Input: part model. Units: mm. Frame: model coordinates. A direction names the side the tool comes from. Round coordinates to 2 decimals unless told otherwise and drop trailing zeros. Write each loop counter-clockwise with the first axis right and the second up, starting at its lowest first coordinate (ties: lowest second). Pieces come first, ordered by that corner, then holes. Notation, with made-up numbers: (77.25, 14) - (92.25, 14) arc R20 ccw to (92.25, 31) - close; hole circle Ø9 at (19.5, -6). An arc over 180 degrees is marked (long way). One line per item, written item: value. Start each with the question number.
```python
from build123d import *

# Parameters (mm, degrees)
BOSS_EXTRUDE1_DEPTH = 25


with BuildPart() as part:
    # Sketch1 → Boss-Extrude1 (new, symmetric)
    with BuildSketch(Plane(origin=(0, 0, 0), x_dir=(0, 0, -1), z_dir=(1, 0, 0))):
        with BuildLine():
            Line((-60, 6.039014916), (60, 6.039014916))
            Line((60, 6.039014916), (60, 30.818764411))
            ThreePointArc((60, 30.818764411), (58.750354063, 32.039014916), (57.500708126, 30.818764411))
            Line((57.500708126, 30.818764411), (57.500708126, 11.039014916))
            ThreePointArc((57.500708126, 11.039014916), (55.57729196, 10.33874836), (53.653875793, 11.039014916))
            Line((53.653875793, 11.039014916), (53.653875793, 22.789014916))
            ThreePointArc((53.653875793, 22.789014916), (52.403875793, 24.039014916), (51.153875793, 22.789014916))
            Line((51.153875793, 22.789014916), (51.153875793, 11.039014916))
            ThreePointArc((51.153875793, 11.039014916), (49.049120778, 10.219058782), (46.944365764, 11.039014916))
            Line((46.944365764, 11.039014916), (46.944365764, 30.818764411))
            ThreePointArc((46.944365764, 30.818764411), (45.694719827, 32.039014916), (44.44507389, 30.818764411))
            Line((44.44507389, 30.818764411), (44.44507389, 11.039014916))
            ThreePointArc((44.44507389, 11.039014916), (42.521657723, 10.33874836), (40.598241557, 11.039014916))
            Line((40.598241557, 11.039014916), (40.598241557, 22.789014916))
            ThreePointArc((40.598241557, 22.789014916), (39.348241557, 24.039014916), (38.098241557, 22.789014916))
            Line((38.098241557, 22.789014916), (38.098241557, 11.039014916))
            ThreePointArc((38.098241557, 11.039014916), (35.993486542, 10.219058782), (33.888731528, 11.039014916))
            Line((33.888731528, 11.039014916), (33.888731528, 30.818764411))
            ThreePointArc((33.888731528, 30.818764411), (32.639085591, 32.039014916), (31.389439654, 30.818764411))
            Line((31.389439654, 30.818764411), (31.389439654, 11.039014916))
            ThreePointArc((31.389439654, 11.039014916), (29.466023487, 10.33874836), (27.54260732, 11.039014916))
            Line((27.54260732, 11.039014916), (27.54260732, 22.789014916))
            ThreePointArc((27.54260732, 22.789014916), (26.29260732, 24.039014916), (25.04260732, 22.789014916))
            Line((25.04260732, 22.789014916), (25.04260732, 11.039014916))
            ThreePointArc((25.04260732, 11.039014916), (22.937852306, 10.219058782), (20.833097291, 11.039014916))
            Line((20.833097291, 11.039014916), (20.833097291, 30.818764411))
            ThreePointArc((20.833097291, 30.818764411), (19.583451354, 32.039014916), (18.333805417, 30.818764411))
            Line((18.333805417, 30.818764411), (18.333805417, 11.039014916))
            ThreePointArc((18.333805417, 11.039014916), (16.410389251, 10.33874836), (14.486973084, 11.039014916))
            Line((14.486973084, 11.039014916), (14.486973084, 22.789014916))
            ThreePointArc((14.486973084, 22.789014916), (13.236973084, 24.039014916), (11.986973084, 22.789014916))
            Line((11.986973084, 22.789014916), (11.986973084, 11.039014916))
            ThreePointArc((11.986973084, 11.039014916), (9.88221807, 10.219058782), (7.777463055, 11.039014916))
            Line((7.777463055, 11.039014916), (7.777463055, 30.818764411))
            ThreePointArc((7.777463055, 30.818764411), (6.527817118, 32.039014916), (5.278171181, 30.818764411))
            Line((5.278171181, 30.818764411), (5.278171181, 11.039014916))
            ThreePointArc((5.278171181, 11.039014916), (3.354755015, 10.33874836), (1.431338848, 11.039014916))
            Line((1.431338848, 11.039014916), (1.431338848, 22.789014916))
            ThreePointArc((1.431338848, 22.789014916), (0.181338848, 24.039014916), (-1.068661152, 22.789014916))
            Line((-1.068661152, 22.789014916), (-1.068661152, 11.039014916))
            ThreePointArc((-1.068661152, 11.039014916), (-3.173416167, 10.219058782), (-5.278171181, 11.039014916))
            Line((-5.278171181, 11.039014916), (-5.278171181, 30.818764411))
            ThreePointArc((-5.278171181, 30.818764411), (-6.527817118, 32.039014916), (-7.777463055, 30.818764411))
            Line((-7.777463055, 30.818764411), (-7.777463055, 11.039014916))
            ThreePointArc((-7.777463055, 11.039014916), (-9.700879222, 10.33874836), (-11.624295388, 11.039014916))
            Line((-11.624295388, 11.039014916), (-11.624295388, 22.789014916))
            ThreePointArc((-11.624295388, 22.789014916), (-12.874295388, 24.039014916), (-14.124295388, 22.789014916))
            Line((-14.124295388, 22.789014916), (-14.124295388, 11.039014916))
            ThreePointArc((-14.124295388, 11.039014916), (-16.229050403, 10.219058782), (-18.333805417, 11.039014916))
            Line((-18.333805417, 11.039014916), (-18.333805417, 30.818764411))
            ThreePointArc((-18.333805417, 30.818764411), (-19.583451354, 32.039014916), (-20.833097291, 30.818764411))
            Line((-20.833097291, 30.818764411), (-20.833097291, 11.039014916))
            ThreePointArc((-20.833097291, 11.039014916), (-22.756513458, 10.33874836), (-24.679929625, 11.039014916))
            Line((-24.679929625, 11.039014916), (-24.679929625, 22.789014916))
            ThreePointArc((-24.679929625, 22.789014916), (-25.929929625, 24.039014916), (-27.179929625, 22.789014916))
            Line((-27.179929625, 22.789014916), (-27.179929625, 11.039014916))
            ThreePointArc((-27.179929625, 11.039014916), (-29.284684639, 10.219058782), (-31.389439654, 11.039014916))
            Line((-31.389439654, 11.039014916), (-31.389439654, 30.818764411))
            ThreePointArc((-31.389439654, 30.818764411), (-32.639085591, 32.039014916), (-33.888731528, 30.818764411))
            Line((-33.888731528, 30.818764411), (-33.888731528, 11.039014916))
            ThreePointArc((-33.888731528, 11.039014916), (-35.812147694, 10.33874836), (-37.735563861, 11.039014916))
            Line((-37.735563861, 11.039014916), (-37.735563861, 22.789014916))
            ThreePointArc((-37.735563861, 22.789014916), (-38.985563861, 24.039014916), (-40.235563861, 22.789014916))
            Line((-40.235563861, 22.789014916), (-40.235563861, 11.039014916))
            ThreePointArc((-40.235563861, 11.039014916), (-42.340318875, 10.219058782), (-44.44507389, 11.039014916))
            Line((-44.44507389, 11.039014916), (-44.44507389, 30.818764411))
            ThreePointArc((-44.44507389, 30.818764411), (-45.694719827, 32.039014916), (-46.944365764, 30.818764411))
            Line((-46.944365764, 30.818764411), (-46.944365764, 11.039014916))
            ThreePointArc((-46.944365764, 11.039014916), (-48.86778193, 10.33874836), (-50.791198097, 11.039014916))
            Line((-50.791198097, 11.039014916), (-50.791198097, 22.789014916))
            ThreePointArc((-50.791198097, 22.789014916), (-52.041198097, 24.039014916), (-53.291198097, 22.789014916))
            Line((-53.291198097, 22.789014916), (-53.291198097, 11.039014916))
            ThreePointArc((-53.291198097, 11.039014916), (-55.395953112, 10.219058782), (-57.500708126, 11.039014916))
            Line((-57.500708126, 11.039014916), (-57.500708126, 30.818764411))
            ThreePointArc((-57.500708126, 30.818764411), (-58.750354063, 32.039014916), (-60, 30.818764411))
            Line((-60, 30.818764411), (-60, 6.039014916))
        make_face()
    extrude(amount=BOSS_EXTRUDE1_DEPTH, both=True)


solid = part.part
```
Q1. Cut plane A-A, the plane y = 13.75. Count the separate pieces of the cut face and the enclosed holes in it, and give its area (3 significant figures).
Q2. Material intervals for probe 1 along Y at (x, z) = (-11, 35.5); probe 2 along Y at (x, z) = (-22, -39.5), sorted ascending. Write a range as from..to.
Q3. Access query for faces 1 (the flat face through (0, 17, -38.098)), 2 (the flat face through (25, 13.4, -12.5)). Directions: +Z, -Z, +X, -X, +Y, -Y. A direction counts if a zero-diameter tool reaches every point of the face in a straight line with its end or side. Return the directions, or none.
Q4. Cut plane D-D, the plane z = -29. Output: boundary loops of the cut face in (x, y).
Q5. Cut plane C-C, the plane z = -49.5. Output: boundary loops of the cut face in (x, y), and give its area (3 significant figures).
Q6. Pull-direction query (Z, two-part tool) for faces 3 (the flat face through (0, 17, 50.791)), 4 (the flat face through (0, 6.039, 1)); classes: pulls with the +Z half, pulls with the -Z half, needs draft (parallel to the pull), parting line crosses it, or undercut.
A:
1. separate pieces: 19
1. enclosed holes: 0
1. area: 2,370 mm²
2. probe 1: y = 6.04..10.36
2. probe 2: y = 6.04..24.03
3. face 1: +X, -X, +Y
3. face 2: +Z, -Z, +X, +Y, -Y
4. outline: (-25, 6.04) - (25, 6.04) - (25, 10.38) - (-25, 10.38) - close
5. outline: (-25, 6.04) - (25, 6.04) - (25, 10.25) - (-25, 10.25) - close
5. area: 211 mm²
6. face 3: undercut
6. face 4: needs draft
